Autodesk Inventor part; units mm, degrees
ref_plane "BODY_DUMMY_XY" through (0, 0, 0) normal (-1, 0, 0) x (0, 0, -1)
ref_plane "BODY_DUMMY_YZ" through (0, 0, 0) normal (0, 0, -1) x (0, -1, 0)
ref_plane "BODY_DUMMY_ZX" through (0, 0, 0) normal (0, -1, 0) x (-1, 0, 0)
sketch "Sketch_13" plane through (0, 0, 0) normal (1, 0, 0) x (0, 1, 0)
  line L0 (16.6132, 20) -> (7, 20)
  line L1 (7, 20) -> (7, 18.4697)
  arc A0 (4, 18.4697) -> (7, 18.4697) centre (5.5, 17) ccw
  line L2 (4, 18.4697) -> (4, 19.5)
  line L3 (4, 19.5) -> (-4, 19.5)
  line L4 (-4, 19.5) -> (-4, 18.4697)
  arc A1 (-7, 18.4697) -> (-4, 18.4697) centre (-5.5, 17) ccw
  line L5 (-7, 18.4697) -> (-7, 20)
  line L6 (-7, 20) -> (-16.6132, 20)
  arc A2 (-16.6132, 20) -> (-20, 16.6132) centre (0, 0) ccw
  line L7 (-20, 16.6132) -> (-20, 7)
  line L8 (-20, 7) -> (-18.4697, 7)
  arc A3 (-18.4697, 4) -> (-18.4697, 7) centre (-17, 5.5) ccw
  line L9 (-18.4697, 4) -> (-19.5, 4)
  line L10 (-19.5, 4) -> (-19.5, -4)
  line L11 (-19.5, -4) -> (-18.4697, -4)
  arc A4 (-18.4697, -7) -> (-18.4697, -4) centre (-17, -5.5) ccw
  line L12 (-18.4697, -7) -> (-20, -7)
  line L13 (-20, -7) -> (-20, -16.6132)
  arc A5 (-20, -16.6132) -> (-16.6132, -20) centre (0, 0) ccw
  line L14 (-16.6132, -20) -> (-7, -20)
  line L15 (-7, -20) -> (-7, -18.4697)
  arc A6 (-4, -18.4697) -> (-7, -18.4697) centre (-5.5, -17) ccw
  line L16 (-4, -18.4697) -> (-4, -19.5)
  line L17 (-4, -19.5) -> (4, -19.5)
  line L18 (4, -19.5) -> (4, -18.4697)
  arc A7 (7, -18.4697) -> (4, -18.4697) centre (5.5, -17) ccw
  line L19 (7, -18.4697) -> (7, -20)
  line L20 (7, -20) -> (16.6132, -20)
  arc A8 (16.6132, -20) -> (20, -16.6132) centre (0, 0) ccw
  line L21 (20, -16.6132) -> (20, -7)
  line L22 (20, -7) -> (18.4697, -7)
  arc A9 (18.4697, -4) -> (18.4697, -7) centre (17, -5.5) ccw
  line L23 (18.4697, -4) -> (19.5, -4)
  line L24 (19.5, -4) -> (19.5, 4)
  line L25 (19.5, 4) -> (18.4697, 4)
  arc A10 (18.4697, 7) -> (18.4697, 4) centre (17, 5.5) ccw
  line L26 (18.4697, 7) -> (20, 7)
  line L27 (20, 7) -> (20, 16.6132)
  arc A11 (20, 16.6132) -> (16.6132, 20) centre (0, 0) ccw
extrude "Extrusion1" add sketch "Sketch_13" along normal blind 72.5
sketch "Sketch_2" plane through (0, 0, 14) normal (0, 0, 1) x (1, 0, 0)
  line L0 (72.5, 14) -> (0, 14)
  line L1 (0, 14) -> (0, 18.5)
  line L2 (0, 18.5) -> (7, 18.5)
  line L3 (7, 18.5) -> (7, 17)
  line L4 (7, 17) -> (7.5415, 16.4585)
  line L5 (7.5415, 16.4585) -> (17, 16.4585)
  line L6 (17, 16.4585) -> (17.1394, 16.7)
  line L7 (17.1394, 16.7) -> (55.3606, 16.7)
  line L8 (55.3606, 16.7) -> (55.5, 16.4585)
  line L9 (55.5, 16.4585) -> (64.9585, 16.4585)
  line L10 (64.9585, 16.4585) -> (65.5, 17)
  line L11 (65.5, 17) -> (65.5, 18.5)
  line L12 (65.5, 18.5) -> (72.5, 18.5)
  line L13 (72.5, 18.5) -> (72.5, 14)
  line L14 (72.5, 14) -> (0, 14)
revolve "Revolution1" cut sketch "Sketch_2" angle 360 about axis through (72.5, 14, 14) along (1, 0, 0)
thread "Thread1"
thread "Thread2"
pattern_linear "Rectangular Pattern1" count 2 spacing 28 along (0, 0, -1) count 2 spacing 28 along (0, -1, 0) of "Revolution1"
sketch "Sketch_5" plane through (0, 0, 0) normal (0, 0, 1) x (1, 0, 0)
  line L0 (61.25, 0) -> (-2, 0)
  line L1 (-2, 0) -> (-2, 6)
  line L2 (-2, 6) -> (16.25, 6)
  line L3 (16.25, 6) -> (16.25, 12.5)
  line L4 (16.25, 12.5) -> (61.25, 12.5)
  line L5 (61.25, 12.5) -> (61.25, 0)
  line L6 (61.25, 0) -> (-2, 0)
revolve "Revolution2" cut sketch "Sketch_5" angle 360 about axis through (61.25, 0, 0) along (1, 0, 0)
sketch "Sketch_4" plane through (0, 0, 0) normal (0, 0, 1) x (1, 0, 0)
  line L0 (9, 13.3066) -> (9, 19.5)
  line L1 (9, 19.5) -> (11.5, 19.5)
  line L2 (11.5, 19.5) -> (11.067, 19.067)
  line L3 (11.067, 19.067) -> (11.067, 14.5)
  line L4 (11.067, 14.5) -> (9, 13.3066)
  line L5 (9, 13.3066) -> (9, 19.5)
revolve "Revolution3" cut sketch "Sketch_4" angle 360 about axis through (9, 13.3066, 0) along (0, -1, 0)
thread "Thread3"
sketch "Sketch_6" plane through (0, 0, 0) normal (0, 0, 1) x (1, 0, 0)
  line L0 (67, 13.3066) -> (67, 19.5)
  line L1 (67, 19.5) -> (69.5, 19.5)
  line L2 (69.5, 19.5) -> (69.067, 19.067)
  line L3 (69.067, 19.067) -> (69.067, 14.5)
  line L4 (69.067, 14.5) -> (67, 13.3066)
  line L5 (67, 13.3066) -> (67, 19.5)
revolve "Revolution4" cut sketch "Sketch_6" angle 360 about axis through (67, 13.3066, 0) along (0, -1, 0)
thread "Thread4"
sketch "Sketch_26" plane through (0, 0, 0) normal (1, 0, 0) x (0, 1, 0)
  circle A0 centre (0, 0) radius 13
  circle A1 centre (0, 0) radius 7.5
extrude "Extrusion2" cut sketch "Sketch_26" along normal blind 2.15
sketch "Sketch_27" plane through (0, 0, 0) normal (1, 0, 0) x (0, 1, 0)
  circle A0 centre (0, 0) radius 7.5
extrude "Extrusion3" cut sketch "Sketch_27" along normal blind 0.5
ref_plane "BODY_DUMMY_XY" through (0, 0, 0) normal (-1, 0, 0) x (0, 0, -1)
ref_plane "BODY_DUMMY_YZ" through (0, 0, 0) normal (0, 0, -1) x (0, -1, 0)
ref_plane "BODY_DUMMY_ZX" through (0, 0, 0) normal (0, -1, 0) x (-1, 0, 0)
ref_plane "BODY_MOUBT1_XY" through (0, 0, 0) normal (-1, 0, 0) x (0, 0, -1)
ref_plane "BODY_MOUBT1_YZ" through (0, 0, 0) normal (0, 0, -1) x (0, -1, 0)
ref_plane "BODY_MOUBT1_ZX" through (0, 0, 0) normal (0, -1, 0) x (-1, 0, 0)
ref_plane "BODY_MOUBT2_XY" through (72.5, 0, 0) normal (1, 0, 0) x (0, 0, -1)
ref_plane "BODY_MOUBT2_YZ" through (72.5, 0, 0) normal (0, 0, -1) x (0, 1, 0)
ref_plane "BODY_MOUBT2_ZX" through (72.5, 0, 0) normal (0, 1, 0) x (1, 0, 0)
ref_plane "BODY_ROD_XY" through (0, 0, 0) normal (-1, 0, 0) x (0, 0, -1)
ref_plane "BODY_ROD_YZ" through (0, 0, 0) normal (0, 0, -1) x (0, -1, 0)
ref_plane "BODY_ROD_ZX" through (0, 0, 0) normal (0, -1, 0) x (-1, 0, 0)
ref_plane "BODY_SWA_XY" through (11, -5.5, 17) normal (-1, 0, 0) x (0, 0, -1)
ref_plane "BODY_SWA_YZ" through (11, -5.5, 17) normal (0, 0, -1) x (0, -1, 0)
ref_plane "BODY_SWA_ZX" through (11, -5.5, 17) normal (0, -1, 0) x (-1, 0, 0)
ref_plane "BODY_SWB_XY" through (63, 5.5, 17) normal (1, 0, 0) x (0, 0, -1)
ref_plane "BODY_SWB_YZ" through (63, 5.5, 17) normal (0, 0, -1) x (0, 1, 0)
ref_plane "BODY_SWB_ZX" through (63, 5.5, 17) normal (0, 1, 0) x (1, 0, 0)
properties part number "CDQSB25-40DM(1_0)_BODY"
Could you check a few things on this model? Use its own coordinates, in mm. A direction names the side the tool comes from. Round coordinates to 2 decimals unless told otherwise and drop trailing zeros. Write each loop counter-clockwise with the first axis right and the second up, starting at its lowest first coordinate (ties: lowest second). Pieces come first, ordered by that corner, then holes. Notation, with made-up numbers: (2.5, 12.25) - (29.5, 12.25) arc R11 ccw to (29.5, 33.25) - close; hole circle Ø11 at (8.5, 32). An arc over 180 degrees is marked (long way). Put each result on its own line as item: value. Start each with the question number.
(1) I want a section at B-B, the plane y = -2.5. Please give me the cut outline in (x, z), plus the area to 3 significant figures.
(2) I need wall thicknesses on probe 1 along Z at (x, y) = (44.5, 14); probe 2 along Z at (x, y) = (12.75, -14); probe 3 along X at (y, z) = (5.5, -3). Which ranges of each line are inside material? Lowest first, please.
(3) For faces 4 (the flat face through (65.5, 15, -17)), 5 (the flat face through (36, 0, -19.5)), 6 (the flat face through (7, -11, -15)), which set-ups out of +Z, -Z, +X, -X, +Y, -Y let a thin tool reach every point of the face, with its end or its side?
(4) I want a section at A-A, the plane x = 19. Give the number of separate pieces and of enclosed holes in the cut face, plus the area to 3 significant figures.
(5) Thinking about a two-plate mould opening in Y: for faces 1 (the flat face through (36, -19.5, 0)), 2 (the flat face through (36, -7, 19)), 3 (the cylindrical face through (35.74, 18.41, -18.36)), which applies, released by +Y, released by -Y, zero draft, split by the parting line, or undercut?
(6) Will these pins go through, and if not, where does the flat tip stop? pin 1 (5.5 mm diameter, centred on y = 14, z = -14, fed in from -X); pin 2 (2 mm diameter, centred on x = 40.5, y = 4, fed in from +Z); pin 3 (4 mm diameter, centred on x = 64.5, y = 2, fed in from -Z).
Here are the results:
1. outline: (0, -19.5) - (72.5, -19.5) - (72.5, 19.5) - (0, 19.5) - (0, 12.76) - (2.15, 12.76) - (2.15, 7.07) - (0.5, 7.07) - (0.5, 5.45) - (16.25, 5.45) - (16.25, 12.25) - (61.25, 12.25) - (61.25, -12.25) - (16.25, -12.25) - (16.25, -5.45) - (0.5, -5.45) - (0.5, -7.07) - (2.15, -7.07) - (2.15, -12.76) - (0, -12.76) - close
1. area: 1,520 mm^2
2. probe 1: z = -20 to -16.7, -11.3 to 11.3, 16.7 to 20
2. probe 2: z = -20 to -16.46, -11.54 to 11.54, 16.46 to 20
2. probe 3: x = 0.5 to 16.25, 61.25 to 72.5
3. face 4: +X
3. face 5: -Z, +X, -X
3. face 6: -X
4. separate pieces: 1
4. enclosed holes: 5
4. area: 843 mm^2
5. face 1: released by -Y
5. face 2: undercut
5. face 3: released by +Y
6. pin 1: stops at x = 7.25
6. pin 2: stops at z = 19.5
6. pin 3: stops at z = -19.5
